Autodesk Inventor part; units mm, degrees
ref_plane "YZ Plane" through (0, 0, 0) normal (1, 0, 0) x (0, 1, 0)
ref_plane "XZ Plane" through (0, 0, 0) normal (0, 1, 0) x (-1, 0, 0)
ref_plane "XY Plane" through (0, 0, 0) normal (0, 0, 1) x (1, 0, 0)
sketch "Boceto1" plane through (0, 0, 0) normal (0, 1, 0) x (-1, 0, 0)
  line L0 (0, 0) -> (0, -70)
  line L1 (0, -70) -> (30, -70)
  line L2 (30, -70) -> (30, -50)
  line L3 (30, -50) -> (12, -39.6077)
  line L4 (12, -24) -> (25, -24)
  line L5 (25, -24) -> (25, -10)
  line L6 (25, -10) -> (8, -10)
  line L7 (8, 0) -> (0, 0)
  line L8 (12, -24) -> (12, -39.6077)
  line L9 (8, -10) -> (8, 0)
  dimension "d0" = 20
  dimension "d1" = 70
  dimension "d2" = 30
  dimension "d5" = 25
  dimension "d6" = 10
  dimension "d7" = 8
  dimension "d8" = 12
  dimension "d9" = 120
  dimension "d10" = 14
extrude "Extrusión1" add sketch "Boceto1" along normal blind 10
equation "\"Radio_pliegue\" = Grosor"
equation "\"Anchura_desahogo_plegado\" = Grosor"
equation "\"Profundidad_desahogo_plegado\" = 0.5 * Grosor"
equation "\"Tamaño_destalonado\" = 4 * Grosor"
equation "\"Remanente_mínimo\" = 2 * Grosor"
equation "\"Radiodetransición\" = Radio_pliegue"
equation "\"Tamaño_de_radio_de_Jacobi\" = Radio_pliegue"
equation "\"TamañoSeparación\" = Grosor"
properties part number "Practica3"
Build history of the part. All positions in model axes, mm. A direction names the side the tool comes from. Coordinates: 2 decimals unless noted, no trailing zeros. Write each loop counter-clockwise with the first axis right and the second up, starting at its lowest first coordinate (ties: lowest second). Pieces come first, ordered by that corner, then holes.
1. Drop flat-ended pins along their axis: pin 1 (3 mm diameter, centred on y = 4.5, z = -18.5, fed in from -X); pin 2 (1 mm diameter, centred on x = -18.5, z = -51.5, fed in from -Y); pin 3 (3 mm diameter, centred on y = 3.5, z = -33.5, fed in from -X); pin 4 (6 mm diameter, centred on x = -23, y = 2.5, fed in from +Z). Give the stop position or say it passes through.
Answer block:
pin 1: stops at x = -25
pin 2: stops at y = 0
pin 3: stops at x = -12
pin 4: stops at z = -10
2. Drill centre lines: probe 1 along X at (y, z) = (3, -7.5); probe 2 along Z at (x, y) = (-8.5, 7); probe 3 along Z at (x, y) = (-14, 7.5). Where is each one in solid material? Low to high.
Answer block:
probe 1: x = -8 to 0
probe 2: z = -70 to -10
probe 3: z = -70 to -40.76, -24 to -10
3. Band-saw the part on D-D, the plane x = -10. Give the cut face in (y, z), and give its area (3 significant figures).
Answer block:
outline: (0, -70) - (10, -70) - (10, -10) - (0, -10) - close
area: 600 mm2
4. Pull direction Z, two halves, no side cores. Call faces 1 (the flat face through (-4, 5, 0)), 2 (the flat face through (-11, 0, -42)), 3 (the flat face through (-18, 5, -24)): released by +Z, released by -Z, zero draft, split by the parting line, or undercut.
Answer block:
face 1: released by +Z
face 2: zero draft
face 3: undercut
5. Band-saw the part on A-A, the plane x = -23.25. Give the cut face in (y, z), and give its area (3 significant figures).
Answer block:
outline: (0, -70) - (10, -70) - (10, -46.1) - (0, -46.1) - close; (0, -24) - (10, -24) - (10, -10) - (0, -10) - close
area: 379 mm2
6. Band-saw the part on B-B, the plane y = 1.5. Give the cut face in (x, z), and give its area (3 significant figures).
Answer block:
outline: (-30, -70) - (0, -70) - (0, 0) - (-8, 0) - (-8, -10) - (-25, -10) - (-25, -24) - (-12, -24) - (-12, -39.61) - (-30, -50) - close
area: 1,440 mm2
7. 3-axis set-ups, long thin cutter, end or side, ignore diameter. For faces 4 (the flat face through (0, 5, -35)), 5 (the flat face through (-21.13, 4.93, -44.88)), 6 (the flat face through (-17, 5, -10)): which of +Z, -Z, +X, -X, +Y, -Y reach the whole face in a straight line?
Answer block:
face 4: +Z, -Z, +X, +Y, -Y
face 5: -X, +Y, -Y
face 6: +Z, -X, +Y, -Y
8. Band-saw the part on C-C, the plane z = -21.5. Give the cut face in (x, y).
Answer block:
outline: (-25, 0) - (0, 0) - (0, 10) - (-25, 10) - close
